Source: CAD feature listing. Evaluate the final solid. Frame: model axes, mm. Face numbers are marked on the shaded views. A direction names the side the tool comes from. Round coordinates to 2 decimals unless told otherwise and drop trailing zeros. Order: outer loops, then holes, each group sorted by start corner. A loop starts at its lowest first (then second) coordinate and runs counter-clockwise, first axis right, second up.
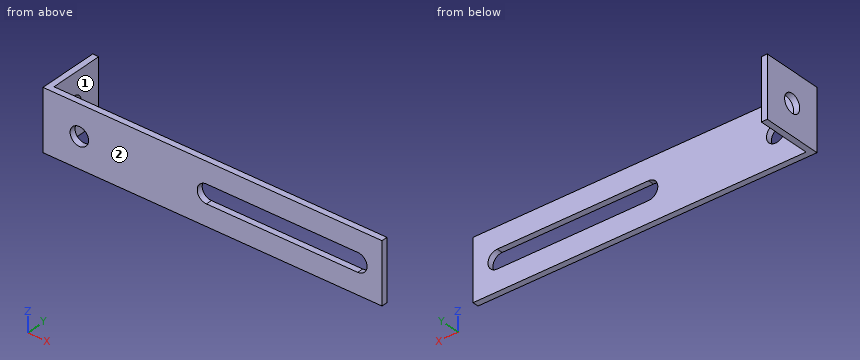
```python
from build123d import *

# Parameters (mm, degrees)
BOSS_EXTRUDE1_DEPTH = 20
SKETCH2_R           = 3.05
CUT_EXTRUDE1_DEPTH  = 116.516232626
SKETCH3_R           = 3.05
CUT_EXTRUDE2_DEPTH  = 116.1868048


with BuildPart() as part:
    # Sketch1 → Boss-Extrude1 (new body)
    with BuildSketch(Plane.XY):
        Polygon((0, 0), (0, 20), (2, 20), (2, 2), (112, 2), (112, 0), align=None)
    extrude(amount=BOSS_EXTRUDE1_DEPTH)

    # Sketch2 → Cut-Extrude1 (cut, through all)
    with BuildSketch(Plane.ZY):
        with Locations((10, 10)):
            Circle(SKETCH2_R)
    extrude(amount=-CUT_EXTRUDE1_DEPTH, mode=Mode.SUBTRACT)

    # Sketch3 → Cut-Extrude2 (cut, through all)
    with BuildSketch(Plane(origin=(0, 2, 0), x_dir=(1, 0, 0), z_dir=(0, 1, 0))):
        with Locations(Location((12, -10, 0), (0, 0, 180))):
            Circle(SKETCH3_R)
        with BuildLine():
            Line((54, -13.05), (104, -13.05))
            ThreePointArc((104, -13.05), (107.05, -10), (104, -6.95))
            Line((104, -6.95), (54, -6.95))
            ThreePointArc((54, -6.95), (50.95, -10), (54, -13.05))
        make_face()
    extrude(amount=-CUT_EXTRUDE2_DEPTH, mode=Mode.SUBTRACT)


solid = part.part
```
1. First-contact query: pin 1 (8 mm diameter, centred on x = 63, z = 4, fed in from +Y); pin 2 (1 mm diameter, centred on y = 5, z = 14, fed in from +X). Flat tips, straight axial feed; report the tip coordinate or a pass-through.
2. Line query: line 1 along Y through (x, z) = (1, 10); line 2 along Y through (x, z) = (83, 18.75). Output: solid intervals per line, ascending.
3. Section D-D on z = 17.25. Return loops of the section in (x, y).
4. Access query for the marked faces 1 and 2. Directions: +Z, -Z, +X, -X, +Y, -Y. A direction counts if a zero-diameter tool reaches every point of the face in a straight line with its end or side. Return the directions, or none.
5. Section A-A on y = 10. Return loops of the section in (x, z).
6. Section B-B on z = 10. Return loops of the section in (x, y).
Result:
1. pin 1: stops at y = 2
1. pin 2: stops at x = 2
2. line 1: y = 0 to 6.95, 13.05 to 20
2. line 2: y = 0 to 2
3. outline: (0, 0) - (112, 0) - (112, 2) - (2, 2) - (2, 20) - (0, 20) - close
4. face 1: +Z, -Z, +X, +Y
4. face 2: +Z, -Z, +X, -X, -Y
5. outline: (0, 0) - (2, 0) - (2, 6.95) - (0, 6.95) - close; (0, 13.05) - (2, 13.05) - (2, 20) - (0, 20) - close
6. outline: (0, 0) - (8.95, 0) - (8.95, 2) - (2, 2) - (2, 6.95) - (0, 6.95) - close; (0, 13.05) - (2, 13.05) - (2, 20) - (0, 20) - close; (15.05, 0) - (50.95, 0) - (50.95, 2) - (15.05, 2) - close; (107.05, 0) - (112, 0) - (112, 2) - (107.05, 2) - close
